from build123d import *

# Parameters (mm, degrees)
F0_R     = 23.2127489618
F1_DEPTH = 105.156
F2_R     = 8.1279313569
F3_DEPTH = 22.098
F4_R     = 8.1619087152
F5_DEPTH = 19.812


with BuildPart() as f1:
    # F0 (on Front) → F1 (new body)
    with BuildSketch(Plane.XZ):
        with Locations((25.789950043, -54.8864603043)):
            Circle(F0_R)
    extrude(amount=-F1_DEPTH)

    # F2 (on face) → F3 (join)
    with BuildSketch(Plane.XZ):
        with BuildLine():
            Line((2.5772010811, 44.0855585039), (2.5772010811, -54.8864603043))
            ThreePointArc((2.5772010811, -54.8864603043), (25.789950043, -31.6737113424), (49.0026990048, -54.8864603043))
            Line((49.0026990048, -54.8864603043), (49.0026990048, 44.0855585039))
            ThreePointArc((49.0026990048, 44.0855585039), (25.789950043, 67.2983074657), (2.5772010811, 44.0855585039))
        make_face()
        with Locations((25.789950043, 44.0855585039)):
            Circle(F2_R, mode=Mode.SUBTRACT)
        with BuildLine():
            ThreePointArc((49.0026990048, -54.8864603043), (25.789950043, -31.6737113424), (2.5772010811, -54.8864603043))
            ThreePointArc((2.5772010811, -54.8864603043), (25.789950043, -78.0992092661), (49.0026990048, -54.8864603043))
        make_face()
        with Locations((25.789950043, -54.8864603043)):
            Circle(F2_R, mode=Mode.SUBTRACT)
    extrude(amount=F3_DEPTH)

    # F4 (on face) → F5 (join)
    with BuildSketch(Plane(origin=(0, 105.156, 0), x_dir=(-1, 0, 0), z_dir=(0, 1, 0))):
        with BuildLine():
            Line((-48.7791649624, 46.4776218361), (-48.7791649624, -51.6727845653))
            ThreePointArc((-48.7791649624, -51.6727845653), (-25.789950043, -31.6737113424), (-2.8007351236, -51.6727845653))
            Line((-2.8007351236, -51.6727845653), (-2.8007351236, 46.4776218361))
            ThreePointArc((-2.8007351236, 46.4776218361), (-25.789950043, 67.2522081192), (-48.7791649624, 46.4776218361))
        make_face()
        with Locations((-25.789950043, 44.144950416)):
            Circle(F4_R, mode=Mode.SUBTRACT)
        with BuildLine():
            ThreePointArc((-2.8007351236, -51.6727845653), (-25.789950043, -31.6737113424), (-48.7791649624, -51.6727845653))
            ThreePointArc((-48.7791649624, -51.6727845653), (-27.4006703184, -78.0432583247), (-2.5772010811, -54.8864603043))
            ThreePointArc((-2.5772010811, -54.8864603043), (-2.6331520225, -53.2757400288), (-2.8007351236, -51.6727845653))
        make_face()
        with Locations((-25.789950043, -54.8864603043)):
            Circle(F4_R, mode=Mode.SUBTRACT)
    extrude(amount=F5_DEPTH)


solid = f1.part
Check sheet for the modelled part. Datum: model origin and axes. Units: mm. A direction names the side the tool comes from. Give positions to 0.01 mm unless a question says otherwise; leave off trailing zeros. Loops run counter-clockwise (first coordinate to the right, second up) from the corner with the lowest first, then second, coordinate; pieces in that order, holes last. Notation, with made-up numbers: M 48.25,4 L 73.25,4 A21 ccw 73.25,27 Z; hole C -1,57.25 d11. An arc over 180 degrees is marked long. Answer as a JSON object with one key per item and string values. Group by question number.
Q1. Cross-section at A-A on z = -21.5. Record the cut outline in (x, y), then the cut area to 3 significant figures.
Q2. Release check for a two-part mould opening along Z. For faces 1 (the cylindrical face through (26.3, -10.894, 67.293)), 2 (the cylindrical face through (29.54, -10.894, 36.875)), 3 (the flat face through (26, 105.156, 9)) record: released by +Z, released by -Z, zero draft, split by the parting line, or undercut.
Q3. Material ranges on line 1 along Z through (x, y) = (26.5, 113.5); line 2 along Y through (x, z) = (47.5, -33.5); line 3 along Y through (x, z) = (22.5, -58), recorded low to high. Write a range as [from, to].
Q4. Cross-section at B-B on x = 24.5. Record the cut outline in (y, z).
Q5. Cross-section at D-D on z = 40.5. Record the cut outline in (x, y), then the cut area to 3 significant figures.
Q6. Access from +Z, -Z, +X, -X, +Y, -Y to the whole of each face (thin tool, end or side, straight path). Record for faces 4 (the flat face through (26, 0, -55)), 5 (the flat face through (26, 105.156, -55)), 6 (the flat face through (2.801, 115, -3)), 7 (the flat face through (48.779, 115, -2)).
Q7. Cross-section at C-C on y = 100. Record the cut outline in (x, z), then the cut area to 3 significant figures.
Q8. Go/stop test with flat-tipped pins: P1, Ø6, axis at y = 113.5, z = -19.5, coming from the -X side; P2, Ø12, axis at y = 79, z = -30, coming from the +X side; P3, Ø13, axis at x = 25.79, z = -54.89, coming from the -Y side. Record where each tip stops, or that it passes through.
Evaluation:
{
 "1": {"outline": "M 2.58,-22.1 L 49,-22.1 L 49,0 L 2.58,0 Z; M 2.8,105.16 L 48.78,105.16 L 48.78,124.97 L 2.8,124.97 Z", "area": "1,940 mm2"},
 "2": {"face 1": "released by +Z", "face 2": "undercut", "face 3": "zero draft"},
 "3": {"line 1": "z = [-78.09, -63.02], [-46.76, 36.01], [52.28, 67.24]", "line 2": "y = [-22.1, 0], [105.16, 124.97]", "line 3": "y = [0, 105.16]"},
 "4": {"outline": "M -22.1,-78.06 L 124.97,-78.06 L 124.97,-62.95 L 105.16,-62.95 L 105.16,-46.83 L 124.97,-46.83 L 124.97,36.09 L 105.16,36.09 L 105.16,-31.71 L 0,-31.71 L 0,36.06 L -22.1,36.06 L -22.1,-46.86 L 0,-46.86 L 0,-62.91 L -22.1,-62.91 Z; M -22.1,52.11 L 0,52.11 L 0,67.26 L -22.1,67.26 Z; M 105.16,52.2 L 124.97,52.2 L 124.97,67.22 L 105.16,67.22 Z"},
 "5": {"outline": "M 2.58,-22.1 L 18.5,-22.1 L 18.5,0 L 2.58,0 Z; M 2.8,105.16 L 18.49,105.16 L 18.49,124.97 L 2.8,124.97 Z; M 33.08,-22.1 L 49,-22.1 L 49,0 L 33.08,0 Z; M 33.09,105.16 L 48.78,105.16 L 48.78,124.97 L 33.09,124.97 Z", "area": "1,330 mm2"},
 "6": {"face 4": "-Y", "face 5": "+Y", "face 6": "+Z, -X, +Y", "face 7": "+Z, +X, +Y"},
 "7": {"outline": "C 25.79,-54.89 d46.43", "area": "1,690 mm2"},
 "8": {"P1": "stops at x = 2.8", "P2": "stops at x = 39.29", "P3": "stops at y = 0"}
}
